Could you check a few things on this model? Use its own coordinates, in mm. Face numbers are marked on the shaded views. A direction names the side the tool comes from. Give positions to 0.01 mm unless a question says otherwise; leave off trailing zeros. Write each loop counter-clockwise with the first axis right and the second up, starting at its lowest first coordinate (ties: lowest second). Pieces come first, ordered by that corner, then holes. Notation, with made-up numbers: M 1.5,-21.75 L 5.5,-21.75 A33 cw 5.5,7.25 Z; hole C 70,71 d7. An arc over 180 degrees is marked long. Write each question's results on one line, items separated by ' | '. Start each with the question number.
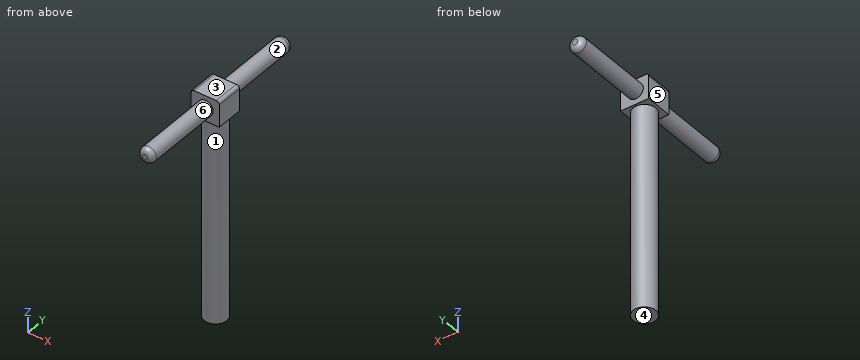
from build123d import *

# Parameters (mm, degrees)
F0_R        = 11.1966523668
F1_DEPTH    = 200
F2_W        = 27.5912405923
F2_H        = 26.4416076243
F3_DEPTH    = 25
F5_R        = 7.5599777125
F6_DEPTH    = 80
F4_R        = 7.5148466093
F7_DEPTH    = 80
F8_T1_DEPTH = 41.4416076243
F9_R        = 5
F10_R       = 5


# Not quite as in the source:
# - a fillet or chamfer that OpenCascade refuses, or shapes differently, is made with other operations: its cross-section is extruded or revolved along the edge and cut away or added
# - a feature names something its author has since deleted; it is built from what else it names


with BuildPart() as f1:
    # F0 (on Top) → F1 (new body)
    with BuildSketch(Plane.XY):
        Circle(F0_R)
    extrude(amount=F1_DEPTH)

    # F2 (on face) → F3 (join)
    with BuildSketch(Plane.XY.offset(200)):
        with Locations((-0.2874094062, 0.0958032906)):
            Rectangle(F2_W, F2_H)
    extrude(amount=F3_DEPTH)

    # F5 (on face) → F6 (join)
    with BuildSketch(Plane(origin=(0, 13.3166071028, 0), x_dir=(-1, 0, 0), z_dir=(0, 1, 0))):
        with Locations((1.2183021754, 212.9181474447)):
            Circle(F5_R)
    extrude(amount=F6_DEPTH)

    # F4 (on face) → F7 (join)
    with BuildSketch(Plane.XZ.offset(13.1250005215)):
        with Locations((0, 212.9505872726)):
            Circle(F4_R)
    extrude(amount=F7_DEPTH)

    # F8: fillet of radius 3 on 2 edges, made by hand

    # F8_s2 → F8_t1 (cut)
    with BuildSketch(Plane.XZ.offset(-20.8166071028)):
        with BuildLine():
            add(Edge.make_bspline(
                [(13.50821089, 222), (13.50821089, 225), (10.50821089, 225)],
                knots=[0, 0, 0, 1, 1, 1], degree=2, weights=[1, 1, 1]))
            Line((10.50821089, 225), (13.50821089, 225))
            Line((13.50821089, 225), (13.50821089, 222))
        make_face()
        with BuildLine():
            add(Edge.make_bspline(
                [(-11.0830297023, 225), (-14.0830297023, 225), (-14.0830297023, 222)],
                knots=[0, 0, 0, 1, 1, 1], degree=2, weights=[1, 1, 1]))
            Line((-14.0830297023, 222), (-14.0830297023, 225))
            Line((-14.0830297023, 225), (-11.0830297023, 225))
        make_face()
    extrude(amount=F8_T1_DEPTH, mode=Mode.SUBTRACT)

    # F9
    f9_edges = [f1.edges().sort_by_distance(p)[0] for p in [
        (6.341676, 93.316607, 212.918147),
    ]]
    fillet(f9_edges, radius=F9_R)

    # F10
    f10_edges = [f1.edges().sort_by_distance(p)[0] for p in [
        (-7.514847, -93.125001, 212.950587),
    ]]
    fillet(f10_edges, radius=F10_R)


solid = f1.part
Q1. If we section it at A-A (z = 51): Please give me the cut outline in (x, y).
Q2. If we section it at B-B (y = 57.5): Please give me the cut outline in (x, z), plus the area to 3 significant figures.
Q3. If we mould it in two halves opening along Z, with no side actions, what happens to the marked faces 1, 2, 3 and 4? For each: pulls with the +Z half, pulls with the -Z half, needs draft (parallel to the pull), parting line crosses it, or undercut.
Q4. For the marked faces 5 and 6, which set-ups out of +Z, -Z, +X, -X, +Y, -Y let a thin tool reach every point of the face, with its end or its side?
Q5. Please list where these lines run through material, in increasing order: line 1 (Y direction, x = 1, z = 164); line 2 (Z direction, x = -10.25, y = 10); line 3 (Y direction, x = -4.25, z = 28.5). Write a range as [from, to].
Q6. I'm going to push flat-ended pins straight in: P1, Ø8, axis at x = -1, y = 69.5, coming from the +Z side; P2, Ø12, axis at x = 4, y = -68.5, coming from the -Z side; P3, Ø12, axis at x = 7.5, z = 162.5, coming from the +Y side. Where does each tip first touch, or does it pass through?
Determined:
1) outline: C 0,0 d22.39
2) outline: C -1.22,212.92 d15.12 | area: 180 mm²
3) face 1: needs draft | face 2: parting line crosses it | face 3: pulls with the +Z half | face 4: pulls with the -Z half
4) face 5: +Z, -Z, -X, +Y, -Y | face 6: -Y
5) line 1: y = [-11.15, 11.15] | line 2: z = [200, 225] | line 3: y = [-10.36, 10.36]
6) P1: stops at z = 220.48 | P2: stops at z = 205.44 | P3: stops at y = 11.1
